Verification items for the finished model (mm, model axes). Face numbers are marked on the shaded views. A direction names the side the tool comes from. Round coordinates to 2 decimals unless told otherwise and drop trailing zeros. Write each loop counter-clockwise with the first axis right and the second up, starting at its lowest first coordinate (ties: lowest second). Pieces come first, ordered by that corner, then holes.
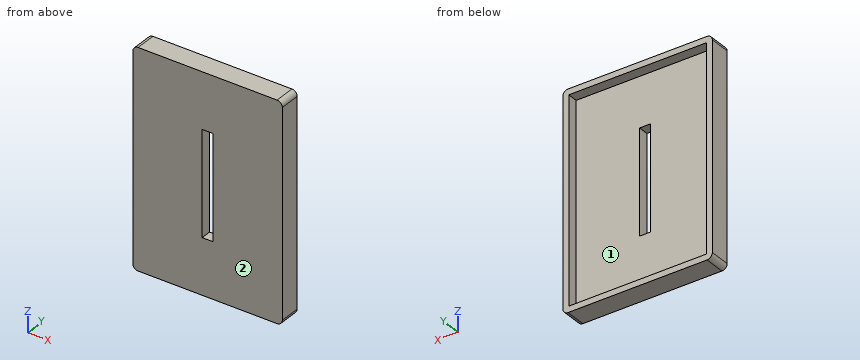
Autodesk Inventor part; units mm, degrees
sketch "Sketch1" plane through (0, 0, 0) normal (0, 1, 0) x (-1, 0, 0)
  line L0 (0, 0) -> (-43, 0)
  line L1 (-43, 0) -> (-43, -62)
  line L2 (-43, -62) -> (0, -62)
  line L3 (0, -62) -> (0, 0)
  dimension "d0" = 43
  dimension "d1" = 62
extrude "Extrusion1" add sketch "Sketch1" along normal blind 3
sketch "Sketch2" plane through (0, 3, 0) normal (0, 1, 0) x (1, 0, 0)
  line L0 (43, 0) -> (43, 62)
  line L1 (0, 0) -> (43, 0)
  line L2 (43, 0) -> (43, 62)
  line L3 (43, 62) -> (0, 62)
  line L4 (0, 62) -> (0, 0)
  line L5 (1.7, 60.3) -> (41.3, 60.3)
  line L6 (41.3, 60.3) -> (41.3, 1.7)
  line L7 (41.3, 1.7) -> (1.7, 1.7)
  line L8 (1.7, 1.7) -> (1.7, 60.3)
  dimension "d4" = 1.7
extrude "Extrusion2" add sketch "Sketch2" along normal blind 3
sketch "Sketch3" plane through (0, 3, 0) normal (0, 1, 0) x (1, 0, 0)
  line L0 (23.05, 46) -> (19.95, 46)
  line L1 (19.95, 46) -> (19.95, 16)
  line L2 (19.95, 16) -> (23.05, 16)
  line L3 (23.05, 16) -> (23.05, 46)
  line L4 (41.3, 60.3) -> (41.3, 1.7)
  line L5 (41.3, 1.7) -> (1.7, 1.7)
  point P0 (0, 0)
  point P1 (41.3, 31)
  point P2 (23.05, 31)
  point P3 (21.5, 1.7)
  point P4 (21.5, 16)
  dimension "d7" = 3.1
  dimension "d8" = 0
  dimension "d9" = 30
  dimension "d15" = 0
extrude "Extrusion3" cut sketch "Sketch3" against normal blind 3
fillet "Fillet1" radius 1.5 4 edges at (43, 3, 0) (0, 3, 0) (0, 3, -62) (43, 3, -62)
equation "\"d0\" = width_inner + 2 * thickness"
equation "\"d1\" = length_inner + 2 * thickness"
equation "\"d2\" = thickness"
equation "\"d5\" = thickness"
equation "\"d7\" = acrylic_thickness"
equation "\"d9\" = acrylic_length"
equation "\"d11\" = thickness"
equation "\"d13\" = 0.5 * thickness"
equation "\"width_inner\" = 37"
equation "\"length_inner\" = 56"
equation "\"thickness\" = 3"
equation "\"acrylic_thickness\" = 3.1"
equation "\"acrylic_length\" = 30"
properties part number "ieee_lid"
Q1. Sectioned sample at C-C (z = -13.5). Enter the section's corners in (x, y), plus the area to 3 significant figures.
Recorded:
outline: (0, 0) - (43, 0) - (43, 6) - (41.3, 6) - (41.3, 3) - (1.7, 3) - (1.7, 6) - (0, 6) - close
area: 139 mm2
Q2. Material ranges on line 1 along X through (y, z) = (2.2, -18.5); line 2 along Z through (x, y) = (36.5, 4.25); line 3 along X through (y, z) = (4.95, -44), recorded low to high.
Recorded:
line 1: x = 0 to 19.95, 23.05 to 43
line 2: z = -62 to -60.3, -1.7 to 0
line 3: x = 0 to 1.7, 41.3 to 43
Q3. Sectioned sample at D-D (x = 40). Enter the section's corners in (y, z), plus the area to 3 significant figures.
Recorded:
outline: (0, -62) - (6, -62) - (6, -60.3) - (3, -60.3) - (3, -1.7) - (6, -1.7) - (6, 0) - (0, 0) - close
area: 196 mm2
Q4. Depth check by flat-ended pin: P1, Ø12, axis at x = 18, z = -41.5, coming from the +Y side. Enter the tip coordinate at first touch or a pass-through.
Recorded:
P1: stops at y = 3
Q5. Sectioned sample at A-A (y = 1.2). Enter the section's corners in (x, z), plus the area to 3 significant figures.
Recorded:
outline: (0, -60.5) arc R1.5 ccw to (1.5, -62) - (41.5, -62) arc R1.5 ccw to (43, -60.5) - (43, -1.5) arc R1.5 ccw to (41.5, 0) - (1.5, 0) arc R1.5 ccw to (0, -1.5) - close; hole (19.95, -46) - (23.05, -46) - (23.05, -16) - (19.95, -16) - close
area: 2,570 mm2
Q6. Tool access check on the marked faces 1 and 2. Record the directions out of +Z, -Z, +X, -X, +Y, -Y that give a thin tool (end or side, any length) a straight path to the whole face; none if there is none.
Recorded:
face 1: +Y
face 2: +Z, -Z, +X, -X, -Y
Q7. Sectioned sample at B-B (z = -23). Enter the section's corners in (x, y).
Recorded:
outline: (0, 0) - (19.95, 0) - (19.95, 3) - (1.7, 3) - (1.7, 6) - (0, 6) - close; (23.05, 0) - (43, 0) - (43, 6) - (41.3, 6) - (41.3, 3) - (23.05, 3) - close
